Read the model definition and answer for the solid it produces. Units are mm, in the model's axes. A direction names the side the tool comes from. Round coordinates to 2 decimals unless told otherwise and drop trailing zeros. Return JSON: item names as keys, results as strings.
from build123d import *

# Parameters (mm, degrees)
SKETCH1_W            = 101.6
SKETCH1_H            = 177.8
BOSS_EXTRUDE2_DEPTH  = 6.35
FILLET1_R            = 15.24
BOSS_EXTRUDE5_DEPTH  = 0.508
CUT_EXTRUDE1_DEPTH   = 0.254
FILLET3_R            = 2.54
FILLET4_R            = 2.54
BOSS_EXTRUDE7_DEPTH  = 1.27
SKETCH6_R            = 5.08
BOSS_EXTRUDE10_DEPTH = 1.27
SKETCH7_R            = 2.54
CUT_EXTRUDE2_DEPTH   = 1.27
CHAMFER1_SIZE        = 1.27
CUT_EXTRUDE6_DEPTH   = 6.35


with BuildPart() as part:
    # Sketch1 → Boss-Extrude2 (new body)
    with BuildSketch(Plane.XY):
        Rectangle(SKETCH1_W, SKETCH1_H)
    extrude(amount=BOSS_EXTRUDE2_DEPTH)

    # Fillet1
    fillet1_edges = [part.edges().sort_by_distance(p)[0] for p in [
        (50.8, -88.9, 3.175),
        (-50.8, -88.9, 3.175),
        (-50.8, 88.9, 3.175),
        (50.8, 88.9, 3.175),
    ]]
    fillet(fillet1_edges, radius=FILLET1_R)

    # Sketch2 → Boss-Extrude5 (add)
    with BuildSketch(Plane.XY):
        with BuildLine():
            Line((12.7, 76.2), (-12.7, 76.2))
            ThreePointArc((-12.7, 76.2), (-16.292102448, 77.687897552), (-17.78, 81.28))
            Line((-17.78, 81.28), (-17.78, 86.36))
            Line((-17.78, 86.36), (-35.56, 86.36))
            ThreePointArc((-35.56, 86.36), (-44.540256121, 82.640256121), (-48.26, 73.66))
            Line((-48.26, 73.66), (-48.26, -73.66))
            ThreePointArc((-48.26, -73.66), (-44.540256121, -82.640256121), (-35.56, -86.36))
            Line((-35.56, -86.36), (35.56, -86.36))
            ThreePointArc((35.56, -86.36), (44.540256121, -82.640256121), (48.26, -73.66))
            Line((48.26, -73.66), (48.26, 73.66))
            ThreePointArc((48.26, 73.66), (44.540256121, 82.640256121), (35.56, 86.36))
            Line((35.56, 86.36), (17.78, 86.36))
            Line((17.78, 86.36), (17.78, 81.28))
            ThreePointArc((17.78, 81.28), (16.292102448, 77.687897552), (12.7, 76.2))
        make_face()
    extrude(amount=-BOSS_EXTRUDE5_DEPTH)

    # Sketch3 → Cut-Extrude1 (cut)
    with BuildSketch(Plane.XY):
        with BuildLine():
            Line((5.08, 81.26519761), (-5.08, 81.26519761))
            ThreePointArc((-5.08, 81.26519761), (-6.35, 82.53519761), (-5.08, 83.80519761))
            Line((-5.08, 83.80519761), (5.08, 83.80519761))
            ThreePointArc((5.08, 83.80519761), (6.35, 82.53519761), (5.08, 81.26519761))
        make_face()
    extrude(amount=CUT_EXTRUDE1_DEPTH, mode=Mode.SUBTRACT)

    # Fillet3
    fillet3_edges = [part.edges().sort_by_distance(p)[0] for p in [
        (0, -88.9, 0),
        (50.8, 0, 0),
        (-50.8, 0, 0),
        (0, 88.9, 0),
        (-46.336307345, 84.436307345, 0),
        (46.336307345, 84.436307345, 0),
        (46.336307345, -84.436307345, 0),
        (-46.336307345, -84.436307345, 0),
    ]]
    fillet(fillet3_edges, radius=FILLET3_R - 0.0001)  # a hair under: the kernel refuses the full size

    # Fillet4
    fillet4_edges = [part.edges().sort_by_distance(p)[0] for p in [
        (0, -88.9, 6.35),
        (-50.8, 0, 6.35),
        (50.8, 0, 6.35),
        (0, 88.9, 6.35),
        (-46.336307345, 84.436307345, 6.35),
        (46.336307345, 84.436307345, 6.35),
        (46.336307345, -84.436307345, 6.35),
        (-46.336307345, -84.436307345, 6.35),
    ]]
    fillet(fillet4_edges, radius=FILLET4_R)

    # Sketch4 → Boss-Extrude7 (add)
    with BuildSketch(Plane.XY.offset(6.35)):
        with BuildLine():
            Line((-12.7, 73.66), (-12.7, 56.173421011))
            ThreePointArc((-12.7, 56.173421011), (-14.931846327, 50.785267338), (-20.32, 48.553421011))
            Line((-20.32, 48.553421011), (-35.56, 48.553421011))
            ThreePointArc((-35.56, 48.553421011), (-40.948153673, 50.785267338), (-43.18, 56.173421011))
            Line((-43.18, 56.173421011), (-43.18, 73.66))
            ThreePointArc((-43.18, 73.66), (-40.948153673, 79.048153673), (-35.56, 81.28))
            Line((-35.56, 81.28), (-20.32, 81.28))
            ThreePointArc((-20.32, 81.28), (-14.931846327, 79.048153673), (-12.7, 73.66))
        make_face()
    extrude(amount=BOSS_EXTRUDE7_DEPTH)

    # Sketch6 → Boss-Extrude10 (add)
    with BuildSketch(Plane.XY.offset(7.62)):
        with Locations(Location((-35.56, 58.713421011, 0), (0, 0, 180))):
            Circle(SKETCH6_R)
        with Locations(Location((-35.56, 71.12, 0), (0, 0, 180))):
            Circle(SKETCH6_R)
    extrude(amount=BOSS_EXTRUDE10_DEPTH)

    # Sketch7 → Cut-Extrude2 (cut)
    with BuildSketch(Plane.XY.offset(7.62)):
        with Locations((-20.32, 64.916710506)):
            Circle(SKETCH7_R)
    extrude(amount=-CUT_EXTRUDE2_DEPTH, mode=Mode.SUBTRACT)

    # Chamfer1
    chamfer1_edges = [part.edges().sort_by_distance(p)[0] for p in [
        (-27.94, 81.28, 7.62),
        (-14.931846327, 79.048153673, 7.62),
        (-12.7, 64.916710506, 7.62),
        (-14.931846327, 50.785267338, 7.62),
        (-27.94, 48.553421011, 7.62),
        (-40.948153673, 50.785267338, 7.62),
        (-43.18, 64.916710506, 7.62),
        (-40.948153673, 79.048153673, 7.62),
    ]]
    chamfer(chamfer1_edges, length=CHAMFER1_SIZE - 0.0001)  # a hair under: the kernel refuses the full size

    # Sketch9 → Cut-Extrude6 (cut)
    with BuildSketch(Plane(origin=(0, -88.9, 0), x_dir=(1, 0, 0), z_dir=(0, 1, 0))):
        with BuildLine():
            Line((5.017161758, -3.762137851), (-5.017161758, -3.762137851))
            ThreePointArc((-5.017161758, -3.762137851), (-5.604299609, -3.175), (-5.017161758, -2.587862149))
            Line((-5.017161758, -2.587862149), (5.017161758, -2.587862149))
            ThreePointArc((5.017161758, -2.587862149), (5.604299609, -3.175), (5.017161758, -3.762137851))
        make_face()
    extrude(amount=CUT_EXTRUDE6_DEPTH, mode=Mode.SUBTRACT)


solid = part.part
Item 1: Straight lines are drawn through the part: L1, parallel to Z at x = -41.5, y = 23; L2, parallel to X at y = 15.5, z = 4; L3, parallel to Y at x = -20.32, z = 6.7. For each, find the intervals that lie inside material, in ascending order. Write a range as [from, to].
Worked answers:
{"L1": "z = [-0.51, 6.35]", "L2": "x = [-50.79, 50.79]", "L3": "y = [48.9, 62.38], [67.46, 80.93]"}
Item 2: A tool of negligible diameter and unlimited length cuts with its end or side. For faces 5 (the cylindrical face through (-44.64, -82.54, -0.25)), 6 (the cylindrical face through (-16.252, 77.649, -0.25)), 7 (the flat face through (0, -86, 3.762)), 8 (the cylindrical face through (-40.405, 57.188, 8.246)), 9 (the cylindrical face through (-44.44, 82.74, -0.25)), from which of +Z, -Z, +X, -X, +Y, -Y can it reach the whole face along a straight path? Write none if from no direction.
Worked answers:
{"face 5": "-Z, -X, -Y", "face 6": "-Z, +Y", "face 7": "-Y", "face 8": "+Z", "face 9": "-Z, -X, +Y"}
Item 3: Flat-ended cylindrical pins translate along their axes: pin 1 (1.9 mm diameter, centred on x = 1, y = -84, fed in from +Z); pin 2 (0.6 mm diameter, centred on y = -32.5, z = -0.5, fed in from -X); pin 3 (3 mm diameter, centred on x = 16.5, z = 0.5, fed in from -Y). Find the tip coordinate at first contact, or state that the pin passes through.
Worked answers:
{"pin 1": "stops at z = 6.35", "pin 2": "stops at x = -48.26", "pin 3": "stops at y = -88.84"}
Item 4: For a pull along Y with two mould halves and no side action, classify faces 1 (the flat face through (-1, 1, -0.508)), 2 (the cylindrical face through (-37.9, 75.63, 8.25)), 3 (the cylindrical face through (-17.974, 63.944, 6.994)), 4 (the cylindrical face through (-46.45, 84.32, 3.18)) as released by +Y, released by -Y, zero draft, split by the parting line, or undercut.
Worked answers:
{"face 1": "zero draft", "face 2": "undercut", "face 3": "undercut", "face 4": "released by +Y"}
